Work out the finished part from the listing and answer in its coordinate system (mm). Coordinates: 2 decimals unless noted, no trailing zeros. Loops run counter-clockwise (first coordinate to the right, second up) from the corner with the lowest first, then second, coordinate; pieces in that order, holes last. Notation, with made-up numbers: (-20, -17.75) -> (39, -17.75) arc R13 cw to (39, -11.75) -> close; hole circle Ø3 at (-14.5, -0.5). An arc over 180 degrees is marked (long way). One line per question, with ' | ' between items.
```python
from build123d import *

# Parameters (mm, degrees)
BOSS_EXTRUDE1_DEPTH = 5.08


with BuildPart() as part:
    # Sketch1 → Boss-Extrude1 (new body)
    with BuildSketch(Plane(origin=(0, 0, 0), x_dir=(1, 0, 0), z_dir=(0, 1, 0))):
        with BuildLine():
            Line((-71.12, 71.12), (-63.5, 71.12))
            Line((-63.5, 71.12), (-63.5, 76.2))
            Line((-63.5, 76.2), (-53.821964394, 76.2))
            Line((-53.821964394, 76.2), (-53.821964394, 68.090455215))
            ThreePointArc((-53.821964394, 68.090455215), (-50.602147322, 64.870638143), (-47.38233025, 68.090455215))
            Line((-47.38233025, 68.090455215), (-47.38233025, 76.2))
            Line((-47.38233025, 76.2), (-28.421964394, 76.2))
            Line((-28.421964394, 76.2), (-28.421964394, 68.090455215))
            ThreePointArc((-28.421964394, 68.090455215), (-25.202147322, 64.870638143), (-21.98233025, 68.090455215))
            Line((-21.98233025, 68.090455215), (-21.98233025, 76.2))
            Line((-21.98233025, 76.2), (-3.021964394, 76.2))
            Line((-3.021964394, 76.2), (-3.021964394, 68.090455215))
            ThreePointArc((-3.021964394, 68.090455215), (0.197852678, 64.870638143), (3.41766975, 68.090455215))
            Line((3.41766975, 68.090455215), (3.41766975, 76.2))
            Line((3.41766975, 76.2), (22.378035606, 76.2))
            Line((22.378035606, 76.2), (22.378035606, 68.090455215))
            ThreePointArc((22.378035606, 68.090455215), (25.597852678, 64.870638143), (28.81766975, 68.090455215))
            Line((28.81766975, 68.090455215), (28.81766975, 76.2))
            Line((28.81766975, 76.2), (47.778035606, 76.2))
            Line((47.778035606, 76.2), (47.778035606, 68.090455215))
            ThreePointArc((47.778035606, 68.090455215), (50.997852678, 64.870638143), (54.21766975, 68.090455215))
            Line((54.21766975, 68.090455215), (54.21766975, 76.2))
            Line((54.21766975, 76.2), (63.5, 76.2))
            Line((63.5, 76.2), (63.5, 71.12))
            Line((63.5, 71.12), (71.12, 71.12))
            Line((71.12, 71.12), (71.12, 63.5))
            Line((71.12, 63.5), (71.12, -63.5))
            Line((71.12, -63.5), (71.12, -71.12))
            Line((71.12, -71.12), (63.5, -71.12))
            Line((63.5, -71.12), (63.5, -76.2))
            Line((63.5, -76.2), (-63.5, -76.2))
            Line((-63.5, -76.2), (-63.5, -71.12))
            Line((-63.5, -71.12), (-71.12, -71.12))
            Line((-71.12, -71.12), (-76.2, -71.12))
            Line((-76.2, -71.12), (-76.2, -63.5))
            Line((-76.2, -63.5), (-76.2, 63.5))
            Line((-76.2, 63.5), (-76.2, 71.12))
            Line((-76.2, 71.12), (-71.12, 71.12))
        make_face()
    extrude(amount=BOSS_EXTRUDE1_DEPTH)


solid = part.part
```
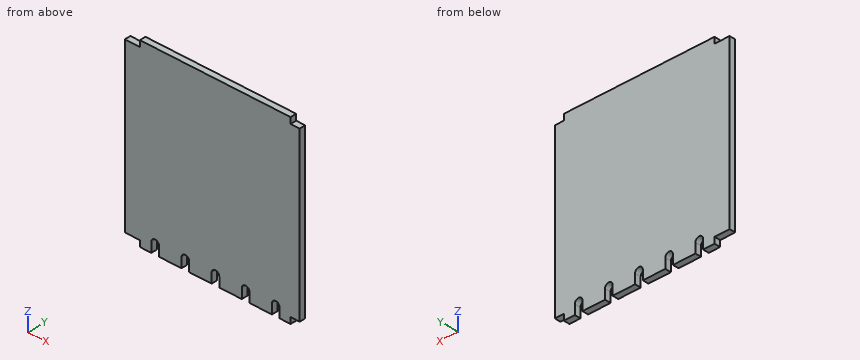
1) Find section B-B (x = -51). Write down the section's boundary in (y, z), plus the area to 3 significant figures.
Check values:
outline: (0, -64.9) -> (5.08, -64.9) -> (5.08, 76.2) -> (0, 76.2) -> close | area: 717 mm^2
2) Find the intervals of material crossed by line 1 along Z through (x, y) = (26, 3.8); line 2 along Z through (x, y) = (-48, 0.4), in increasing order.
Check values:
line 1: z = -64.9 to 76.2 | line 2: z = -66.19 to 76.2
3) Flat-ended cylindrical pins translate along their axes: pin 1 (1.5 mm diameter, centred on x = -70.5, y = 3, fed in from -Z); pin 2 (2.5 mm diameter, centred on y = 4, z = 74.5, fed in from -X); pin 3 (2 mm diameter, centred on x = 1, y = 4.5, fed in from -Z). Find the tip coordinate at first contact, or state that the pin passes through.
Check values:
pin 1: stops at z = -71.12 | pin 2: stops at x = -63.5 | pin 3: stops at z = -65.42
